Check sheet for the modelled part. Datum: model origin and axes. Units: mm. Face numbers are marked on the shaded views. Give positions to 0.01 mm unless a question says otherwise; leave off trailing zeros. Order: outer loops, then holes, each group sorted by start corner. A loop starts at its lowest first (then second) coordinate and runs counter-clockwise, first axis right, second up.
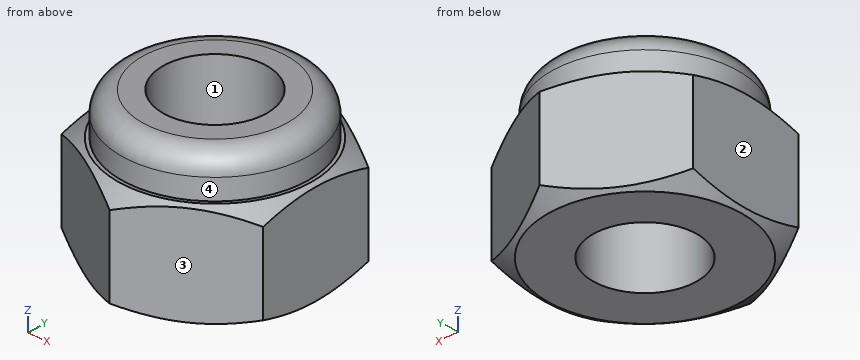
from build123d import *

# Parameters (mm, degrees)
F0_R     = 1.5
F1_DEPTH = 3
F4_W     = 1.2
F4_H     = 1.2
F6_R     = 0.6


with BuildPart() as f1:
    # F0 (on Top) → F1 (new body)
    with BuildSketch(Plane.XY):
        Polygon((2.925, -1.68875), (2.925, 1.68875), (0, 3.377499), (-2.925, 1.68875), (-2.925, -1.68875), (0, -3.377499), align=None)
        Circle(F0_R, mode=Mode.SUBTRACT)
    extrude(amount=F1_DEPTH)

    # F2 (on Front) → F3 (revolve, cut)
    with BuildSketch(Plane.XZ):
        Polygon((4.878461, 3), (2.8, 3), (4.878461, 1.8), align=None)
        Polygon((2.8, 0), (4.878461, 0), (4.878461, 1.2), align=None)
    revolve(axis=Axis((0, 0, 1.5), (0, 0, 1)), mode=Mode.SUBTRACT)

    # F4 (on Front) → F5 (revolve)
    with BuildSketch(Plane.XZ):
        with Locations((2.1, 3.6)):
            Rectangle(F4_W, F4_H)
    revolve(axis=Axis((0, 0, 1.5), (0, 0, 1)))

    # F6
    f6_edges = [f1.edges().sort_by_distance(p)[0] for p in [
        (-2.7, 0, 4.2),
    ]]
    fillet(f6_edges, radius=F6_R)


solid = f1.part
1) Draft check along Y on the marked faces 1, 2, 3 and 4. Enter one of: +Y half, -Y half, draft (parallel to the pull), parting line (faces both ways), or undercut.
Recorded:
face 1: undercut
face 2: draft
face 3: -Y half
face 4: parting line
2) Material ranges on L1, parallel to Y at x = 0, z = 3.3; L2, parallel to Z at x = 2.35, y = 1.75; L3, parallel to Y at x = -0.85, z = 0.6, recorded low to high.
Recorded:
L1: y = -2.7 to -1.5, 1.5 to 2.7
L2: z = 0.08 to 2.92
L3: y = -2.89 to -1.24, 1.24 to 2.89
3) Section check A-A, the plane y = 0. Record the cut outline in (x, z) (3 decimals), then the cut area to 3 significant figures.
Recorded:
outline: (-2.925, 0.072) - (-2.8, 0) - (-1.5, 0) - (-1.5, 4.2) - (-2.1, 4.2) arc R0.6 ccw to (-2.7, 3.6) - (-2.7, 3) - (-2.8, 3) - (-2.925, 2.928) - close; (1.5, 0) - (2.8, 0) - (2.925, 0.072) - (2.925, 2.928) - (2.8, 3) - (2.7, 3) - (2.7, 3.6) arc R0.6 ccw to (2.1, 4.2) - (1.5, 4.2) - close
area: 11.3 mm2
4) Section check B-B, the plane z = 3.45. Record the cut outline in (x, y).
Recorded:
outline: circle Ø5.4 at (0, 0); hole circle Ø3 at (0, 0)
